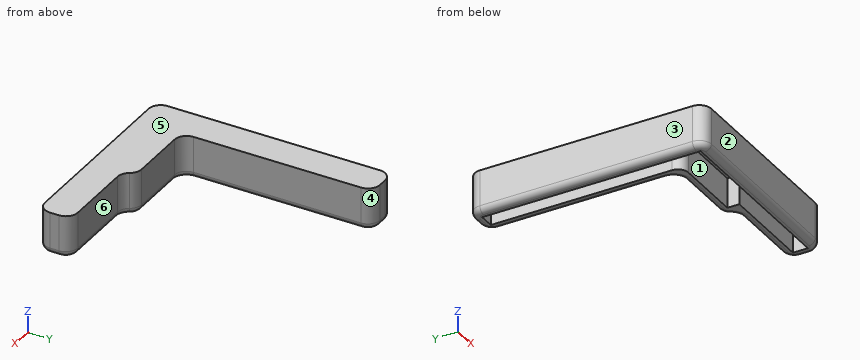
Autodesk Inventor part; units mm, degrees
ref_plane "YZ Plane" through (0, 0, 0) normal (1, 0, 0) x (0, 1, 0)
ref_plane "XZ Plane" through (0, 0, 0) normal (0, 1, 0) x (-1, 0, 0)
ref_plane "XY Plane" through (0, 0, 0) normal (0, 0, 1) x (1, 0, 0)
sketch "Skizze1" plane through (0, 0, 0) normal (0, 0, 1) x (1, 0, 0)
  line L0 (-2, -29) -> (-2, -31) construction
  line L1 (0, -31) -> (-2, -31) construction
  line L2 (-2, -29) -> (0, -29) construction
  line L3 (0, -31) -> (26.4999, -31) construction
  line L4 (28.4999, -31) -> (26.4999, -31) construction
  line L5 (26.4999, -29) -> (28.4999, -29) construction
  line L6 (28.4999, -31) -> (28.4999, -29) construction
  line L7 (26.4999, -29) -> (0, -29) construction
  line L8 (13, -27) -> (13, -29) construction
  line L9 (13, -27) -> (2, -27) construction
  arc A0 (0, -25) -> (2, -27) centre (2, -25) ccw construction
  arc A1 (-2, -25) -> (2, -29) centre (2, -25) ccw construction
  line L10 (-2, 0) -> (-2, -25) construction
  line L11 (0, -25) -> (0, 0) construction
  line L12 (-2, 0) -> (-2, 5) construction
  line L13 (0, 5) -> (0, 0) construction
  line L14 (0, 5) -> (-2, 5) construction
  line L15 (28.4999, -31) -> (-2, -31) construction
  line L16 (-2, -31) -> (-2, 5) construction
  line L17 (-2, 5) -> (0, 5) construction
  line L18 (0, 5) -> (0, -25) construction
  arc A2 (0, -25) -> (2, -27) centre (2, -25) ccw construction
  line L19 (2, -27) -> (13, -27) construction
  line L20 (13, -27) -> (13, -29) construction
  line L21 (13, -29) -> (28.4999, -29) construction
  line L22 (28.4999, -31) -> (28.4999, -29) construction
  line L23 (-2.25, 5.25) -> (-2.25, -31.25)
  line L24 (-2.25, -31.25) -> (28.7499, -31.25)
  line L25 (28.7499, -31.25) -> (28.7499, -28.75)
  line L26 (28.7499, -28.75) -> (13.25, -28.75)
  line L27 (13.25, -28.75) -> (13.25, -26.75)
  line L28 (13.25, -26.75) -> (2, -26.75)
  arc A3 (0.25, -25) -> (2, -26.75) centre (2, -25) ccw
  line L29 (0.25, -25) -> (0.25, 5.25)
  line L30 (0.25, 5.25) -> (-2.25, 5.25)
  line L31 (-3.75, -30.75) -> (-3.75, 4.75)
  line L32 (-1.75, 6.75) -> (-0.25, 6.75)
  line L33 (1.75, 4.75) -> (1.75, -23.25)
  arc A4 (1.75, -25) -> (2, -25.25) centre (2, -25) ccw
  line L34 (3.75, -25.25) -> (13.2859, -25.25)
  line L35 (14.75, -25.25) -> (14.75, -25.25)
  line L36 (16.75, -27.25) -> (28.2499, -27.25)
  line L37 (30.2499, -29.25) -> (30.2499, -30.75)
  line L38 (28.2499, -32.75) -> (-1.75, -32.75)
  arc A5 (28.2499, -32.75) -> (30.2499, -30.75) centre (28.2499, -30.75) ccw
  arc A6 (30.2499, -29.25) -> (28.2499, -27.25) centre (28.2499, -29.25) ccw
  arc A7 (-3.75, -30.75) -> (-1.75, -32.75) centre (-1.75, -30.75) ccw
  arc A8 (15.0179, -26.25) -> (16.75, -27.25) centre (16.75, -25.25) ccw
  arc A9 (15.0179, -26.25) -> (13.2859, -25.25) centre (13.2859, -27.25) ccw
  arc A10 (1.75, -23.25) -> (3.75, -25.25) centre (3.75, -23.25) ccw
  arc A11 (1.75, 4.75) -> (-0.25, 6.75) centre (-0.25, 4.75) ccw
  arc A12 (-1.75, 6.75) -> (-3.75, 4.75) centre (-1.75, 4.75) ccw
  dimension "d0" = 0.25
  dimension "d1" = 1.5
  dimension "d2" = 2
  dimension "d3" = 2
extrude "Extrusion1" add sketch "Skizze1" against normal blind 5
fillet "Rundung1" radius 1 15 edges at (-3.1642, -32.1642, -5) (-3.75, -13, -5) (-3.1642, 6.1642, -5) (-1, 6.75, -5) (1.1642, 6.1642, -5) (1.75, -9.25, -5) (2.3358, -24.6642, -5) (8.5179, -25.25, -5) (14.2859, -25.5179, -5) (15.75, -26.9821, -5) (22.5, -27.25, -5) (29.6641, -27.8358, -5) (30.2499, -30, -5) (29.6641, -32.1642, -5) (13.25, -32.75, -5)
sketch "Skizze2" plane through (0, 0, 0) normal (0, 0, 1) x (1, 0, 0)
  line L0 (28.7499, -31.25) -> (-2.25, -31.25)
  line L1 (-2.25, -31.25) -> (-2.25, 5.25)
  line L2 (-2.25, 5.25) -> (0.25, 5.25)
  line L3 (0.25, 5.25) -> (0.25, -25)
  arc A0 (0.25, -25) -> (2, -26.75) centre (2, -25) ccw
  line L4 (2, -26.75) -> (13.25, -26.75)
  line L5 (13.25, -26.75) -> (13.25, -28.75)
  line L6 (13.25, -28.75) -> (28.7499, -28.75)
  line L7 (28.7499, -28.75) -> (28.7499, -31.25)
  line L8 (30.2499, -30.75) -> (30.2499, -29.25)
  arc A1 (30.2499, -29.25) -> (28.2499, -27.25) centre (28.2499, -29.25) ccw
  line L9 (28.2499, -27.25) -> (16.75, -27.25)
  arc A2 (15.0179, -26.25) -> (16.75, -27.25) centre (16.75, -25.25) ccw
  arc A3 (15.0179, -26.25) -> (13.2859, -25.25) centre (13.2859, -27.25) ccw
  line L10 (13.2859, -25.25) -> (3.75, -25.25)
  arc A4 (1.75, -23.25) -> (3.75, -25.25) centre (3.75, -23.25) ccw
  line L11 (1.75, -23.25) -> (1.75, 4.75)
  arc A5 (1.75, 4.75) -> (-0.25, 6.75) centre (-0.25, 4.75) ccw
  line L12 (-0.25, 6.75) -> (-1.75, 6.75)
  arc A6 (-1.75, 6.75) -> (-3.75, 4.75) centre (-1.75, 4.75) ccw
  line L13 (-3.75, 4.75) -> (-3.75, -30.75)
  arc A7 (-3.75, -30.75) -> (-1.75, -32.75) centre (-1.75, -30.75) ccw
  line L14 (-1.75, -32.75) -> (28.2499, -32.75)
  arc A8 (28.2499, -32.75) -> (30.2499, -30.75) centre (28.2499, -30.75) ccw
  point P0 (0, 0)
extrude "Extrusion2" add sketch "Skizze2" along normal blind 2 contours L0 L1 L2 L3 A0 L4 L5 L6 L7 | A8 L14 A7 L13 A6 L12 A5 L11 A4 L10 A3 A2 L9 A1 L8
properties part number "Stand_Vorne"
Read the model definition and answer for the solid it produces. Units are mm, in the model's axes. Face numbers are marked on the shaded views. A direction names the side the tool comes from. Coordinates: 2 decimals unless noted, no trailing zeros. Loops run counter-clockwise (first coordinate to the right, second up) from the corner with the lowest first, then second, coordinate; pieces in that order, holes last.
Q1. Each of these flat-tipped pins is pushed along its axis until it touches: pin 1 Ø3 at (x, z) = (8, -0.5) entering from +Y; pin 2 Ø4 at (y, z) = (-18, -2) entering from +X; pin 3 Ø1 at (y, z) = (-26, 1) entering from +X. Where does it stop, or does it pass through?
Q2. The part is cut by section B-B on z = -2. Write down the section's boundary in (x, y).
Q3. Consider probe 1 along X at (y, z) = (-8, -1.5); probe 2 along Y at (x, z) = (-1.5, -2.75); probe 3 along Y at (x, z) = (26.5, -0.75). Determine where each line is inside the solid, lowest interval first.
Q4. The part is cut by section A-A on x = 9.5. Write down the section's boundary in (y, z).
Q5. The mould has two halves that part along Y. Classify the marked faces 1, 2, 3 and 4: +Y half, -Y half, draft (parallel to the pull), parting line (faces both ways), or undercut.
Q6. The part is cut by section C-C on y = -13. Write down the section's boundary in (x, z).
Q7. Which of the six approach directions +Z, -Z, +X, -X, +Y, -Y give full straight-line access (tool end or side, diameter ignored) to the marked faces 5 and 6?
Results below:
1. pin 1: stops at y = -25.25
1. pin 2: stops at x = 1.75
1. pin 3: stops at x = 15.19
2. outline: (-3.75, -30.75) arc R2 ccw to (-1.75, -32.75) - (28.25, -32.75) arc R2 ccw to (30.25, -30.75) - (30.25, -29.25) arc R2 ccw to (28.25, -27.25) - (16.75, -27.25) arc R2 cw to (15.02, -26.25) arc R2 ccw to (13.29, -25.25) - (3.75, -25.25) arc R2 cw to (1.75, -23.25) - (1.75, 4.75) arc R2 ccw to (-0.25, 6.75) - (-1.75, 6.75) arc R2 ccw to (-3.75, 4.75) - close; hole (-2.25, -31.25) - (28.75, -31.25) - (28.75, -28.75) - (13.25, -28.75) - (13.25, -26.75) - (2, -26.75) arc R1.75 cw to (0.25, -25) - (0.25, 5.25) - (-2.25, 5.25) - close
3. probe 1: x = -3.75 to -2.25, 0.25 to 1.75
3. probe 2: y = -32.75 to -31.25, 5.25 to 6.75
3. probe 3: y = -32.75 to -31.25, -28.75 to -27.25
4. outline: (-32.75, -4) arc R1 ccw to (-31.75, -5) - (-31.25, -5) - (-31.25, 0) - (-26.75, 0) - (-26.75, -5) - (-26.25, -5) arc R1 ccw to (-25.25, -4) - (-25.25, 2) - (-32.75, 2) - close
5. face 1: undercut
5. face 2: -Y half
5. face 3: draft
5. face 4: +Y half
6. outline: (-3.75, -4) arc R1 ccw to (-2.75, -5) - (-2.25, -5) - (-2.25, 0) - (0.25, 0) - (0.25, -5) - (0.75, -5) arc R1 ccw to (1.75, -4) - (1.75, 2) - (-3.75, 2) - close
7. face 5: +Z, +X, -X, +Y, -Y
7. face 6: +Z, -Z, +X, +Y
